Part model, mm, in its own coordinate system. Face numbers are marked on the shaded views. Round coordinates to 2 decimals unless told otherwise and drop trailing zeros. Order: outer loops, then holes, each group sorted by start corner. A loop starts at its lowest first (then second) coordinate and runs counter-clockwise, first axis right, second up. Notation, with made-up numbers: (40.5, 89) -> (80.5, 89) arc R27 cw to (80.5, 106) -> close; hole circle Ø5 at (-39, -1). An arc over 180 degrees is marked (long way). Return JSON: item names as keys, results as strings. Group by question number.
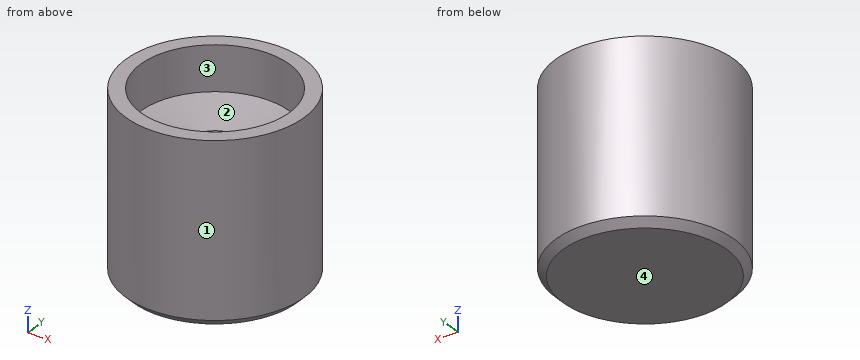
from build123d import *

# Parameters (mm, degrees)
SKETCH2_R           = 6
BOSS_EXTRUDE1_DEPTH = 12
CHAMFER1_SIZE       = 0.1
CHAMFER1_SIZE2      = 0.123280305
CHAMFER2_SIZE       = 0.5


with BuildPart() as part:
    # Sketch2 → Boss-Extrude1 (new body)
    with BuildSketch(Plane.XY):
        Circle(SKETCH2_R)
    extrude(amount=BOSS_EXTRUDE1_DEPTH)

    # Sketch3 → Cut-Revolve1 (revolve, cut)
    with BuildSketch(Plane(origin=(0, 0, 0), x_dir=(1, 0, 0), z_dir=(0, 1, 0))):
        Polygon((0, -12), (0, -3.5), (1.5, -3.5), (1.5, -8.382855568), (5, -9), (5, -12), align=None)
    revolve(axis=Axis((0, 0, 12), (0, 0, -1)), mode=Mode.SUBTRACT)

    # Chamfer1
    chamfer1_edges = [part.edges().sort_by_distance(p)[0] for p in [
        (-1.5, 0, 8.382855568),
    ]]
    chamfer1_side = [part.faces().sort_by_distance(p)[0] for p in [
        (-3.25, 0, 8.691427784),
    ]]
    chamfer(chamfer1_edges, length=CHAMFER1_SIZE, length2=CHAMFER1_SIZE2, reference=chamfer1_side[0])

    # Chamfer2
    chamfer2_edges = [part.edges().sort_by_distance(p)[0] for p in [
        (-6, 0, 0),
    ]]
    chamfer(chamfer2_edges, length=CHAMFER2_SIZE)


solid = part.part
(1) Saw through at A-A, the plane z = 5.25. List the corners of the cut face in (x, y).
(2) Mould opens along Y. For the marked faces 1, 2, 3 and 4 say: pulls with the +Y half, pulls with the -Y half, needs draft (parallel to the pull), parting line crosses it, or undercut.
(3) Pin check, flat tips, straight feed: P1, Ø1.5, axis at x = -1, y = 3.5, coming from the -Z side; P2, Ø1.5, axis at x = 3, z = 2, coming from the +Y side; P3, Ø1.5, axis at x = -2, z = 3.5, coming from the -Y side; P4, Ø2, axis at x = 4, z = 3, coming from the +Y side. Stop position of each tip, or through.
(4) Probe L1, parallel to Y at x = 0, z = 11.3; L2, parallel to Y at x = 0, z = 7.35; L3, parallel to Z at x = 0.5, y = 0.75. List the from-to ranges inside material, lowest first. Write a range as [from, to].
Results are:
{
 "1": {"outline": "circle Ø12 at (0, 0); hole circle Ø3 at (0, 0)"},
 "2": {"face 1": "parting line crosses it", "face 2": "undercut", "face 3": "undercut", "face 4": "needs draft"},
 "3": {"P1": "stops at z = 0", "P2": "stops at y = 5.56", "P3": "stops at y = -5.87", "P4": "stops at y = 5.2"},
 "4": {"L1": "y = [-6, -5], [5, 6]", "L2": "y = [-6, -1.5], [1.5, 6]", "L3": "z = [0, 3.5]"}
}
